from build123d import *

# Parameters (mm, degrees)
PAD_DEPTH    = 10
SKETCH001_R  = 1.5
PAD001_DEPTH = 10


with BuildPart() as part:
    # Sketch → Pad (new body)
    with BuildSketch(Plane.XY):
        Polygon((66.116543, 0), (0, 0), (42.261826, 90.630779), (51.324904, 86.404596), (15.696856, 10), (66.116543, 10), align=None)
    extrude(amount=PAD_DEPTH)

    # Sketch001 (on Face4 of Pad) → Pad001 (join)
    with BuildSketch(Plane(origin=(9.063078, -4.226183, 0), x_dir=(0.422618, 0.906308, 0), z_dir=(0.906308, -0.422618, 0))):
        with BuildLine():
            Line((100, 10), (90, 10))
            Line((90, 10), (90, 20))
            ThreePointArc((100, 20), (95, 25), (90, 20))
            Line((100, 10), (100, 20))
        make_face()
        with Locations((95, 20)):
            Circle(SKETCH001_R, mode=Mode.SUBTRACT)
        with BuildLine():
            Line((35, 10), (35, 20))
            ThreePointArc((35, 20), (30, 25), (25, 20))
            Line((25, 10), (25, 20))
            Line((35, 10), (25, 10))
        make_face()
        with Locations((30, 20)):
            Circle(SKETCH001_R, mode=Mode.SUBTRACT)
    extrude(amount=-PAD001_DEPTH)


solid = part.part
Can you work these out from the model? Positions are in its coordinate system, mm. A direction names the side the tool comes from. Give positions to 0.01 mm unless a question says otherwise; leave off trailing zeros. Order: outer loops, then holes, each group sorted by start corner. A loop starts at its lowest first (then second) coordinate and runs counter-clockwise, first axis right, second up. Notation, with made-up numbers: M 44,-38.5 L 63,-38.5 A36 ccw 63,-4.5 Z; hole C -4,36.5 d7. An arc over 180 degrees is marked long. Use a Markdown table: item, result. Add a question column.
Item 1: Suppose I cut it at C-C (z = 7). List the corners of the cut face in (x, y) for me.
Item 2: If I drill on L1, parallel to Z at x = 37, y = 78; L2, parallel to Y at x = 47.5, z = 7.5, over which ranges is the centre line in solid material (lowest first)? Write a range as [from, to].
Item 3: For faces 1 (the flat face through (33.76, 48.74, 4.93)), 2 (the flat face through (42.631, 79.425, 14.93)), 3 (the flat face through (19.387, 29.578, 14.93)), which set-ups out of +Z, -Z, +X, -X, +Y, -Y let a thin tool reach every point of the face, with its end or its side?
Item 4: Suppose I cut it at A-A (z = 14.5). List the corners of the cut face in (x, y) for me, then the cut area to 3 significant figures.
Item 5: We'd pull the mould along Z, two halves only. Please class faces 4 (the cylindrical face through (17.878, 26.343, 20.451)), 5 (the flat face through (21.712, 22.9, 17.605)), 6 (the cylindrical face through (17.3, 25.1, 25)): +Z half, -Z half, draft (parallel to the pull), parting line (faces both ways), or undercut.
Item 6: Will these pins go through, and if not, where does the flat tip stop? pin 1 (4 mm diameter, centred on x = 25, z = 4.5, fed in from +Y); pin 2 (8 mm diameter, centred on x = 10.5, z = 16.5, fed in from -Y); pin 3 (12 mm diameter, centred on x = 22, z = 11.5, fed in from +Y).
Item 7: Suppose I cut it at D-D (x = 46). Count the separate pieces of the cut face and the enclosed holes in it, then the cut area to 3 significant figures.
Item 8: Suppose I cut it at B-B (x = 25.5). List the corners of the cut face in (y, z) for me, then the cut area to 3 significant figures.
Answer sheet:
| question | item | result |
|---|---|---|
| 1 | outline | M 0,0 L 66.12,0 L 66.12,10 L 15.7,10 L 51.32,86.4 L 42.26,90.63 Z |
| 2 | L1 | z = [0, 10] |
| 2 | L2 | y = [0, 10], [78.2, 88.19] |
| 3 | face 1 | +Z, -Z, +X |
| 3 | face 2 | +Z, -X, -Y |
| 3 | face 3 | +Z, +X, +Y |
| 4 | outline | M 10.57,22.66 L 19.63,18.43 L 23.85,27.49 L 14.79,31.72 Z; M 38.04,81.57 L 47.1,77.34 L 51.32,86.4 L 42.26,90.63 Z |
| 4 | area | 200 mm² |
| 5 | face 4 | undercut |
| 5 | face 5 | draft |
| 5 | face 6 | +Z half |
| 6 | pin 1 | stops at y = 57.9 |
| 6 | pin 2 | stops at y = 20.82 |
| 6 | pin 3 | stops at y = 59.64 |
| 7 | separate pieces | 2 |
| 7 | enclosed holes | 1 |
| 7 | area | 385 mm² |
| 8 | outline | M 0,0 L 10,0 L 10,10 L 0,10 Z; M 31.02,0 L 54.68,0 L 54.68,10 L 31.02,10 Z |
| 8 | area | 337 mm² |
